Geometry check sheet. Reference: the model listing, model coordinates, mm. A direction names the side the tool comes from. Give positions to 0.01 mm unless a question says otherwise; leave off trailing zeros. Order: outer loops, then holes, each group sorted by start corner. A loop starts at its lowest first (then second) coordinate and runs counter-clockwise, first axis right, second up. Notation, with made-up numbers: M 59,0.5 L 108,0.5 A15 ccw 108,5.5 Z; hole C -21.75,35 d5. An arc over 180 degrees is marked long. Answer as CSV lines item,"result". Start each with the question number.
Autodesk Inventor part; units mm, degrees
ref_plane "YZ Plane" through (0, 0, 0) normal (1, 0, 0) x (0, 1, 0)
ref_plane "XZ Plane" through (0, 0, 0) normal (0, 1, 0) x (-1, 0, 0)
ref_plane "XY Plane" through (0, 0, 0) normal (0, 0, 1) x (1, 0, 0)
sketch "Sketch1" plane through (0, 0, 0) normal (1, 0, 0) x (0, 1, 0)
  line L0 (-2.5, 10) -> (2.5, 10)
  line L1 (2.5, 10) -> (2.5, -10)
  line L2 (2.5, -10) -> (-2.5, -10)
  line L3 (-2.5, -10) -> (-2.5, 10)
  line L4 (-2.5, 10) -> (2.5, -10) construction
  line L5 (2.5, 10) -> (-2.5, -10) construction
  point P0 (0, 0)
  dimension "d0" = 5
  dimension "d1" = 20
extrude "Extrusion1" add sketch "Sketch1" along normal blind 17
sketch "Sketch3" plane through (0, -2.5, 10) normal (0, 0, 1) x (1, 0, 0)
  line L0 (3, 5) -> (0, 5)
  line L1 (0, 5) -> (0, 15)
  line L2 (0, 15) -> (3, 15)
  line L3 (3, 15) -> (3, 5)
  point P0 (0, 2.5)
  dimension "d8" = 3
  dimension "d9" = 10
extrude "Extrusion3" add sketch "Sketch3" against normal up to surface (20 mm away)
sketch "Sketch4" plane through (0, 0, 0) normal (-1, 0, 0) x (0, 0, 1)
  circle A0 centre (-121.4441, 7.5) radius 2
  circle A1 centre (-132.4441, 7.5) radius 2
  point P0 (0, 0)
extrude "Extrusion4" cut sketch "Sketch4" against normal through all
sketch "Sketch5" plane through (0, 0, 0) normal (-1, 0, 0) x (0, 0, 1)
  line L0 (-2.5, -37.5) -> (-2.5, -2.5)
  line L1 (-10, -2.5) -> (10, -2.5)
  line L2 (2.5, -2.5) -> (2.5, -37.5)
  line L3 (2.5, -37.5) -> (-2.5, -37.5)
  point P0 (0, 0)
extrude "Extrusion5" add sketch "Sketch5" against normal blind 5
sketch "Sketch6" plane through (0, 0, 0) normal (-1, 0, 0) x (0, 0, 1)
  circle A0 centre (-5.5, 7.5) radius 2
  circle A1 centre (5.5, 7.5) radius 2
  point P0 (0, 0)
extrude "Extrusion6" cut sketch "Sketch6" against normal blind 10
ref_plane "Work Plane1" through (0, -2.5, -10) normal (0, -1, 0) x (1, 0, 0)
split_face "Split1"
sketch "Sketch7" plane through (0, -2.5, 2.5) normal (-1, 0, 0) x (0, 0, 1)
  line L0 (-12.5, 5) -> (7.5, 5)
  line L1 (-5, 0) -> (0, 0)
  line L2 (7.5, 0) -> (0, 0)
  line L3 (7.5, 15) -> (7.5, 0)
  line L4 (7.5, 15) -> (-12.5, 15)
  line L5 (-12.5, 0) -> (-12.5, 15)
  line L6 (-5, 0) -> (-12.5, 0)
  circle A0 centre (3, 10) radius 2
  circle A1 centre (-8, 10) radius 2
  line L7 (-5, 0) -> (0, 0)
  line L8 (-5, 0) -> (-5, -35)
  line L9 (-5, -35) -> (0, -35)
  line L10 (0, -35) -> (0, 0)
  point P0 (-2.5, 2.5)
extrude "Extrusion7" add sketch "Sketch7" along normal blind 4 contours L0 L3 L2 L1 L6 L5 | L1 L10 L9 L8
sketch "Sketch8" plane through (5, 0, 0) normal (1, 0, 0) x (0, 0, -1)
  line L0 (-2.5, -2.5) -> (-2.5, -37.5)
  line L1 (-2.5, -37.5) -> (2.5, -37.5)
  line L2 (2.5, -37.5) -> (2.5, -2.5)
  line L3 (-2.5, -2.5) -> (2.5, -2.5)
  point P0 (0, 0)
extrude "Extrusion8" cut sketch "Sketch8" against normal blind 4
move faces "Move1" translate (-0.5, 0, 0) faces at (-4, -14.1667, 0.8333)
fillet "Fillet3" radius 2 6 edges at (6.25, -2.5, -10) (17, -2.5, 0) (6.25, -2.5, 10) (-4.5, 0, 10) (-4.5, 2.5, 0) (-4.5, 0, -10)
fillet "Fillet4" radius 2 4 edges at (-4.5, -2.5, 5.25) (-3.9142, -1.9142, 9.4142) (-4.5, -2.5, -5.25) (-3.9142, -1.9142, -9.4142)
sketch "Sketch11" plane through (15, -2.5, -8) normal (0, -1, 0) x (1, 0, 0)
  point P0 (-15, 8)
sketch "Sketch2" plane through (17, 0, 0) normal (1, 0, 0) x (0, 0, -1)
  line L0 (-2.4746, -2.5) -> (2.5254, -2.5)
  line L1 (2.5254, -2.5) -> (2.5254, -37.5)
  line L2 (2.5254, -37.5) -> (-2.4746, -37.5)
  line L3 (-2.4746, -37.5) -> (-2.4746, -2.5)
  line L4 (-10, -2.5) -> (10, -2.5)
  line L5 (2.5254, -2.5) -> (2.5254, 0)
  line L6 (-2.4746, -2.5) -> (-2.4746, -0.5)
  line L7 (10, -0.5) -> (-10, -0.5)
  line L8 (2.5254, 0) -> (-2.2155, 0)
  line L9 (-2.4746, -0.5) -> (-2.4746, 0)
  line L10 (-2.4746, 0) -> (-2.1408, 0)
  point P0 (0, 0)
  dimension "d4" = 5
  dimension "d5" = 35
sketch "Sketch12" plane through (15, -2.5, -8) normal (0, -1, 0) x (1, 0, 0)
  point P0 (-15, 8)
properties part number "reverse_finger"
Item 1: Section check D-D on z = -2. Record the boundary of the cut face in (x, y), then the cut area to 3 significant figures.
Item 2: Section check B-B on y = 7.5. Record the boundary of the cut face in (x, z).
Item 3: Draft check along Y on faces 1 (the face through (1.479, 9.483, 5.24)), 2 (the face through (1, -20, 0)), 3 (the face through (-3.93, -1.9, -5.21)), 4 (the face through (1.479, 9.483, -5.76)). Enter one of: pulls with the +Y half, pulls with the -Y half, needs draft (parallel to the pull), parting line crosses it, or undercut.
Item 4: Scan lines: line 1 along Y through (x, z) = (15, -6.75); line 2 along Y through (x, z) = (2.1, 5.5); line 3 along Y through (x, z) = (2.5, -4.75). Record each from-to range of solid material in increasing order.
Item 5: Depth check by flat-ended pin: pin 1 Ø8 at (y, z) = (9, 3) entering from +X; pin 2 Ø10 at (x, z) = (14, 3) entering from -Y; pin 3 Ø6 at (x, y) = (4, 7) entering from -Z; pin 4 Ø3 at (x, z) = (-2, 0) entering from +Y. Enter the tip coordinate at first touch or a pass-through.
Item 6: Section check C-C on x = 1.5. Record the boundary of the cut face in (y, z), then the cut area to 3 significant figures.
Item 7: Access from +Z, -Z, +X, -X, +Y, -Y to the whole of each face (thin tool, end or side, straight path). Record for faces 5 (the face through (-3.63, 0.65, 9.65)), 6 (the face through (-3.93, -1.9, 5.29)), 7 (the face through (3, 8, 0)), 8 (the face through (0, 7, 0)), 9 (the face through (-4.5, -17, 0)).
Item 8: Section check A-A on z = -5.5. Record the boundary of the cut face in (x, y).
Numbers:
1,outline,"M -4.5,-37.5 L 1,-37.5 L 1,-2.5 L 15,-2.5 A2 ccw 17,-0.5 L 17,2.5 L 3,2.5 L 3,12.5 L 0,12.5 L 0,2.5 L -2.5,2.5 A2 ccw -4.5,0.5 Z"
1,area,"328 mm2"
2,outline,"M 0,-10 L 3,-10 L 3,-7.5 L 0,-7.5 Z; M 0,-3.5 L 3,-3.5 L 3,3.5 L 0,3.5 Z; M 0,7.5 L 3,7.5 L 3,10 L 0,10 Z"
3,face 1,"undercut"
3,face 2,"needs draft"
3,face 3,"pulls with the -Y half"
3,face 4,"undercut"
4,line 1,"-2.5 to 2.5"
4,line 2,"-2.5 to 5.5, 9.5 to 12.5"
4,line 3,"-2.5 to 5.65, 9.35 to 12.5"
5,pin 1,"x = 3"
5,pin 2,"y = -2.5"
5,pin 3,"z = -10"
5,pin 4,"y = 2.5"
6,outline,"M -2.5,-8 A2 ccw -0.5,-10 L 12.5,-10 L 12.5,10 L -0.5,10 A2 ccw -2.5,8 Z; hole C 7.5,-5.5 d4; hole C 7.5,5.5 d4"
6,area,"273 mm2"
7,face 5,"+Z, -X, +Y, -Y"
7,face 6,"+Z, -X, -Y"
7,face 7,"+Z, -Z, +X, +Y"
7,face 8,"+Z, -Z, -X, +Y"
7,face 9,"+Z, -Z, -X, +Y, -Y"
8,outline,"M -4.5,-0.5 A2 ccw -2.5,-2.5 L 15,-2.5 A2 ccw 17,-0.5 L 17,2.5 L 3,2.5 L 3,5.5 L 0,5.5 L 0,2.5 L -2.5,2.5 A2 ccw -4.5,0.5 Z; M 0,9.5 L 3,9.5 L 3,12.5 L 0,12.5 Z"
